```python
from build123d import *

# Parameters (mm, degrees)
BOSS_EXTRUDE1_DEPTH = 6.35
SKETCH6_R           = 3.760114337
CUT_EXTRUDE3_DEPTH  = 12.7
SKETCH8_R           = 3.81
CUT_EXTRUDE4_DEPTH  = 2.54


with BuildPart() as part:
    # Sketch1 → Boss-Extrude1 (new body, symmetric)
    with BuildSketch(Plane(origin=(0, 0, 0), x_dir=(0, 0, -1), z_dir=(1, 0, 0))):
        Polygon((0, 0), (0, -17.874529582), (2.54, -17.874529582), (2.54, 2.445470418), (-12.7, 2.445470418), (-12.7, 0), align=None)
    extrude(amount=BOSS_EXTRUDE1_DEPTH, both=True)

    # Sketch6 → Cut-Extrude3 (cut)
    with BuildSketch(Plane(origin=(0, 0, -2.54), x_dir=(-1, 0, 0), z_dir=(0, 0, -1))):
        with Locations((0, -7.714529582)):
            Circle(SKETCH6_R)
    extrude(amount=-CUT_EXTRUDE3_DEPTH, mode=Mode.SUBTRACT)

    # Sketch8 → Cut-Extrude4 (cut)
    with BuildSketch(Plane(origin=(0, 2.445470418, 0), x_dir=(1, 0, 0), z_dir=(0, 1, 0))):
        with Locations((0, -5.08)):
            Circle(SKETCH8_R)
    extrude(amount=-CUT_EXTRUDE4_DEPTH, mode=Mode.SUBTRACT)


solid = part.part
```
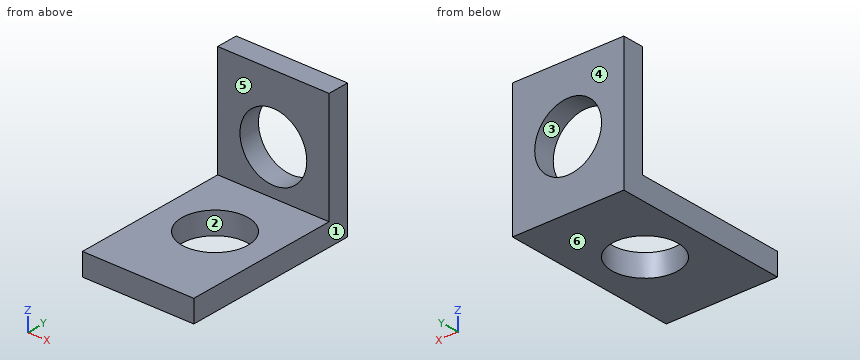
Here's how the part is built. I have some questions about the finished solid (model axes, mm). Face numbers are marked on the shaded views. A direction names the side the tool comes from. Coordinates: 2 decimals unless noted, no trailing zeros. Loops run counter-clockwise (first coordinate to the right, second up) from the corner with the lowest first, then second, coordinate; pieces in that order, holes last. Notation, with made-up numbers: (-8, 43) -> (6, 43) arc R18 ccw to (6, 57) -> close; hole circle Ø3 at (-11, -36). An arc over 180 degrees is marked (long way). Return JSON: item names as keys, results as strings.
1) For the marked faces 5 and 6, which set-ups out of +Z, -Z, +X, -X, +Y, -Y let a thin tool reach every point of the face, with its end or its side?
Results below:
{"face 5": "+Z, +X, -X, -Y", "face 6": "-Z, +X, -X, +Y, -Y"}
2) I need wall thicknesses on line 1 (Y direction, x = 0, z = -1.1); line 2 (Z direction, x = 0, y = 1.8); line 3 (Y direction, x = 5.5, z = 5.25). Which ranges of each line are inside material? Lowest first, please. Write a range as from..to.
Results below:
{"line 1": "-17.87..-11.47, -3.95..2.45", "line 2": "-2.54..1.27, 8.89..12.7", "line 3": "0..2.45"}
3) If we section it at C-C, the plane y = -4.25: Write out the boundary of the cut face in (x, z), then the cut area to 3 significant figures.
Results below:
{"outline": "(-6.35, -2.54) -> (-1.46, -2.54) -> (-1.46, 0) -> (-6.35, 0) -> close; (1.46, -2.54) -> (6.35, -2.54) -> (6.35, 0) -> (1.46, 0) -> close", "area": "24.8 mm²"}
4) If we section it at B-B, the plane z = 5.08: Write out the boundary of the cut face in (x, y).
Results below:
{"outline": "(-6.35, 0) -> (-3.81, 0) -> (-3.81, 2.45) -> (-6.35, 2.45) -> close; (3.81, 0) -> (6.35, 0) -> (6.35, 2.45) -> (3.81, 2.45) -> close"}
5) If we section it at D-D, the plane x = 5.75: Write out the boundary of the cut face in (y, z).
Results below:
{"outline": "(-17.87, -2.54) -> (2.45, -2.54) -> (2.45, 12.7) -> (0, 12.7) -> (0, 0) -> (-17.87, 0) -> close"}
6) If we section it at A-A, the plane x = 0: Write out the boundary of the cut face in (y, z).
Results below:
{"outline": "(-17.87, -2.54) -> (-11.47, -2.54) -> (-11.47, 0) -> (-17.87, 0) -> close; (-3.95, -2.54) -> (2.45, -2.54) -> (2.45, 1.27) -> (0, 1.27) -> (0, 0) -> (-3.95, 0) -> close; (0, 8.89) -> (2.45, 8.89) -> (2.45, 12.7) -> (0, 12.7) -> close"}
7) Will these pins go through, and if not, where does the flat tip stop? pin 1 (5 mm diameter, centred on y = -4.5, z = 5.5, fed in from -X); pin 2 (6 mm diameter, centred on x = 1, y = -7, fed in from +Z); pin 3 (6 mm diameter, centred on x = -3.5, y = -2.5, fed in from +Z); pin 4 (4 mm diameter, centred on x = -2, z = 5, fed in from -Y).
Results below:
{"pin 1": "through", "pin 2": "z = 0", "pin 3": "z = 12.7", "pin 4": "y = 0"}
8) Thinking about a two-plate mould opening in X: for the marked faces 1, 2, 3 and 4, which applies, +X half, -X half, draft (parallel to the pull), parting line (faces both ways), or undercut?
Results below:
{"face 1": "+X half", "face 2": "undercut", "face 3": "undercut", "face 4": "draft"}
